```python
from build123d import *

# Parameters (mm, degrees)
SCALE1_SCALE = 0.168


with BuildPart() as part:
    # Sketch1 → Revolve1 (revolve)
    with BuildSketch(Plane.XY, mode=Mode.PRIVATE) as revolve1_sk:
        with BuildLine():
            Line((-19.243896498, 37), (-12.688168408, 37))
            ThreePointArc((-12.688168408, 37), (-3.743896498, 33), (5.200375412, 37))
            Line((5.200375412, 37), (11.756103502, 37))
            Line((11.756103502, 37), (11.756103502, 27.1))
            ThreePointArc((11.756103502, 27.1), (11.141027743, 25.61507576), (9.656103502, 25))
            Line((9.656103502, 25), (-17.143896498, 25))
            ThreePointArc((-17.143896498, 25), (-18.628820738, 25.61507576), (-19.243896498, 27.1))
            Line((-19.243896498, 27.1), (-19.243896498, 37))
        make_face()
    revolve(revolve1_sk.sketch.rotate(Axis((-29.974665728, 0, 0), (1, 0, 0)), 90), axis=Axis((-29.974665728, 0, 0), (1, 0, 0)))


with BuildPart() as part_1:
    # Scale1: scaled about (-3.743896498, 0, 0)
    add(part.part.scale(SCALE1_SCALE).moved(Location((-3.114921886, 0, 0))))


solid = part_1.part
```
The model under review builds one solid part; all positions refer to its coordinate system, in mm. Give positions to 0.01 mm unless a question says otherwise; leave off trailing zeros. Write each loop counter-clockwise with the first axis right and the second up, starting at its lowest first coordinate (ties: lowest second). Pieces come first, ordered by that corner, then holes. Notation, with made-up numbers: M 46.5,-35 L 83.5,-35 A12 ccw 83.5,-19 Z; hole C -40,46.5 d9. An arc over 180 degrees is marked long. Answer in a Markdown table with one row per item.
Item 1: Add section D-D on x = -3.9. Give the boundary of the cut face in (y, z).
Check sheet entries:
| item | result |
|---|---|
| outline | C 0,0 d11.1; hole C 0,0 d8.4 |
Item 2: Add section A-A on z = 0. Give the boundary of the cut face in (x, y).
Check sheet entries:
| item | result |
|---|---|
| outline | M -6.35,-6.22 L -5.25,-6.22 A2.02 cw -2.24,-6.22 L -1.14,-6.22 L -1.14,-4.55 A0.35 ccw -1.49,-4.2 L -6,-4.2 A0.35 ccw -6.35,-4.55 Z; M -6.35,4.55 A0.35 ccw -6,4.2 L -1.49,4.2 A0.35 ccw -1.14,4.55 L -1.14,6.22 L -2.24,6.22 A2.02 cw -5.25,6.22 L -6.35,6.22 Z |
Item 3: Add section C-C on x = -5.8. Give the boundary of the cut face in (y, z), plus the area to 3 significant figures.
Check sheet entries:
| item | result |
|---|---|
| outline | C 0,0 d12.43; hole C 0,0 d8.4 |
| area | 66.0 mm2 |
Item 4: For P1, Ø3, axis at x = -2, z = 4, coming from the -Y side, flat-tipped, find the tip position at first contact; note if it passes through.
Check sheet entries:
| item | result |
|---|---|
| P1 | y = -5.69 |
Item 5: For line 1 along Y through (x, z) = (-4.45, 0); line 2 along Z through (x, y) = (-4.1, 3); line 3 along Y through (x, z) = (-5.05, 0), list the stretches that pass through material, from the lowest coordinate up.
Check sheet entries:
| item | result |
|---|---|
| line 1 | -5.67 to -4.2, 4.2 to 5.67 |
| line 2 | -4.7 to -2.94, 2.94 to 4.7 |
| line 3 | -6.02 to -4.2, 4.2 to 6.02 |
Item 6: Draft analysis for pull direction Z (two halves, no side actions). For faces 1 (the face through (-1.68, -0.27, -6.21)), 2 (the face through (-1.14, -5, 0)), 3 (the face through (-3.775, -1.262, 4.006)), state which applies: +Z half, -Z half, draft (parallel to the pull), parting line (faces both ways), or undercut.
Check sheet entries:
| item | result |
|---|---|
| face 1 | parting line |
| face 2 | draft |
| face 3 | undercut |
